CAD build for the part. Positions are in the model's coordinates, mm. A direction names the side the tool comes from. Coordinates: 2 decimals unless noted, no trailing zeros. Loops run counter-clockwise (first coordinate to the right, second up) from the corner with the lowest first, then second, coordinate; pieces in that order, holes last. Notation, with made-up numbers: (42.25, -5.5) -> (101.25, -5.5) arc R22 cw to (101.25, 9.5) -> close; hole circle Ø3 at (61, -24). An arc over 180 degrees is marked (long way). Write each question's results on one line, items separated by ' | '.
from build123d import *

# Parameters (mm, degrees)
BOSS_EXTRUDE1_DEPTH     = 25
FILLET1_R               = 19.05
CUT_EXTRUDE1_DEPTH      = 74.437759365
CUT_EXTRUDE1_DEPTH_BACK = 74.437759365
SKETCH3_R               = 14.5
SKETCH3_W               = 14.2875
SKETCH3_H               = 12.7
SKETCH5_R               = 4.8895
CUT_EXTRUDE2_DEPTH      = 12.7


with BuildPart() as part:
    # Sketch2 → Boss-Extrude1 (new, symmetric)
    with BuildSketch(Plane.XY):
        Polygon((-28.936184536, 20), (15.526994141, -43.5), (53.626994141, -43.5), (9.163815464, 20), align=None)
    extrude(amount=BOSS_EXTRUDE1_DEPTH, both=True)

    # Fillet1
    fillet1_edges = [part.edges().sort_by_distance(p)[0] for p in [
        (-9.886184536, 20, 25),
        (-9.886184536, 20, -25),
    ]]
    fillet(fillet1_edges, radius=FILLET1_R)

    # Sketch3 → Cut-Extrude1 (cut, two sides: drawn at the far end of the back side and taken through both)
    with BuildSketch(Plane(origin=(0, 0, 0), x_dir=(0, 0, -1), z_dir=(1, 0, 0)).offset(-CUT_EXTRUDE1_DEPTH_BACK)):
        with Locations(Location((0, 0, 0), (0, 0, 270))):
            Circle(SKETCH3_R)
        with Locations((0, -32.07)):
            Rectangle(SKETCH3_W, SKETCH3_H)
    extrude(amount=CUT_EXTRUDE1_DEPTH + CUT_EXTRUDE1_DEPTH_BACK, mode=Mode.SUBTRACT)

    # Sketch5 → Cut-Extrude2 (cut)
    with BuildSketch(Plane.XZ.offset(43.5)):
        with Locations((34.576994141, 0)):
            Circle(SKETCH5_R)
    extrude(amount=-CUT_EXTRUDE2_DEPTH, mode=Mode.SUBTRACT)


solid = part.part
1) Pin check, flat tips, straight feed: pin 1 (7 mm diameter, centred on x = 38.5, z = 3, fed in from +Y); pin 2 (5 mm diameter, centred on y = -1, z = -10.5, fed in from +X); pin 3 (9 mm diameter, centred on x = 34.58, z = 0, fed in from +Y); pin 4 (12 mm diameter, centred on x = 40.5, y = -15.5, fed in from -Z). Stop position of each tip, or through.
Outcome:
pin 1: stops at y = -16.9 | pin 2: passes through | pin 3: stops at y = -13.89 | pin 4: stops at z = -25
2) Drill centre lines: L1, parallel to Z at x = 4.5, y = -26; L2, parallel to Z at x = -1, y = 0; L3, parallel to Y at x = 12.5, z = 4.5. Where is each one in solid material? Low to high. Write a range as from..to.
Outcome:
L1: z = -25..-7.14, 7.14..25 | L2: z = -25..-14.5, 14.5..25 | L3: y = -39.18..-38.42, -25.72..-13.78, 13.78..15.24
3) Slice it at B-B (x = 18). Write the cut outline in (y, z), then the cut area to 3 significant figures.
Outcome:
outline: (-43.5, -25) -> (0.95, -25) arc R19.05 ccw to (7.38, -23.88) -> (7.38, -12.48) arc R14.5 cw (long way) to (7.38, 12.48) -> (7.38, 23.88) arc R19.05 ccw to (0.95, 25) -> (-43.5, 25) -> close; hole (-38.42, -7.14) -> (-25.72, -7.14) -> (-25.72, 7.14) -> (-38.42, 7.14) -> close | area: 1,820 mm^2
4) Slice it at A-A (y = -1.5). Write the cut outline in (x, z).
Outcome:
outline: (-13.88, -25) -> (24.22, -25) -> (24.22, -14.42) -> (-13.88, -14.42) -> close; (-13.88, 14.42) -> (24.22, 14.42) -> (24.22, 25) -> (-13.88, 25) -> close
5) Which spindle directions (+Z, -Z, +X, -X, +Y, -Y) get a long thin tool onto all of the face, cutting with end or side? Do faces 4 (the flat face through (26, -32, 7.144)), 5 (the flat face through (19, -21, 25)). Say none if no direction does.
Outcome:
face 4: +X, -X | face 5: +Z, +X, -X, +Y, -Y
6) Slice it at C-C (z = 0). Write the cut outline in (x, y), then the cut area to 3 significant figures.
Outcome:
outline: (-28.94, 20) -> (-25.09, 14.5) -> (13.01, 14.5) -> (9.16, 20) -> close; (-4.78, -14.5) -> (3.08, -25.72) -> (41.18, -25.72) -> (33.32, -14.5) -> close; (11.97, -38.42) -> (15.53, -43.5) -> (29.69, -43.5) -> (29.69, -38.42) -> close; (39.47, -43.5) -> (53.63, -43.5) -> (50.07, -38.42) -> (39.47, -38.42) -> close | area: 781 mm^2
7) Slice it at D-D (x = 44.5). Write the cut outline in (y, z).
Outcome:
outline: (-43.5, -25) -> (-30.47, -25) -> (-30.47, -7.14) -> (-38.42, -7.14) -> (-38.42, 7.14) -> (-30.47, 7.14) -> (-30.47, 25) -> (-43.5, 25) -> close
8) Two-plate mould, pull along Y, no slides. Class faces 1 (the cylindrical face through (39.094, -40.996, -1.873)), 2 (the flat face through (30.75, -38.42, 3.28)), 3 (the flat face through (36.647, -19.25, 0.35)): pulls with the +Y half, pulls with the -Y half, needs draft (parallel to the pull), parting line crosses it, or undercut.
Outcome:
face 1: needs draft | face 2: undercut | face 3: pulls with the +Y half
